Could you check a few things on this model? Use its own coordinates, in mm. A direction names the side the tool comes from. Give positions to 0.01 mm unless a question says otherwise; leave off trailing zeros. Loops run counter-clockwise (first coordinate to the right, second up) from the corner with the lowest first, then second, coordinate; pieces in that order, holes last. Notation, with made-up numbers: M 58,81.5 L 77,81.5 A33 ccw 77,113.5 Z; hole C 18,38 d1. An arc over 180 degrees is marked long. Return JSON: item names as keys, results as strings. Group by question number.
1. If we section it at A-A (z = 33): Write out the boundary of the cut face in (x, y), plus the area to 3 significant figures.
2. Please list where these lines run through material, in increasing order: line 1 (X direction, y = -131.5, z = 76); line 2 (Y direction, x = -170.5, z = 73); line 3 (Y direction, x = -2.5, z = 38.5).
3. For faces 1 (the flat face through (47.709, -113, 50)), 2 (the flat face through (-113, 50.8, 50)), which set-ups out of +Z, -Z, +X, -X, +Y, -Y let a thin tool reach every point of the face, with its end or its side?
4. For pin 1 (5 mm diameter, centred on y = -47, z = 81.5, fed in from -X); pin 2 (8 mm diameter, centred on x = -108, z = 40.5, fed in from -Y); pin 3 (8 mm diameter, centred on y = 23, z = 20.5, fed in from +X), each with a flat end and sliding along its axis, tell me the tip position at first contact or that it passes through.
5. If we section it at C-C (x = -16): Write out the boundary of the cut face in (y, z).
6. If we section it at B-B (y = -64.5): Write out the boundary of the cut face in (x, z).
```python
from build123d import *

# Parameters (mm, degrees)
F1_DEPTH = 101.6
F2_DEPTH = 152.4
F3_DEPTH = 152.4


with BuildPart() as f1:
    # F0 (on Top) → F1 (new body)
    with BuildSketch(Plane.XY):
        with BuildLine():
            Line((50.8, -73.0918422341), (50.8, 0))
            ThreePointArc((50.8, 0), (35.9210244843, 35.9210244843), (0, 50.8))
            Line((0, 50.8), (-76.0997384787, 50.8))
            Line((-76.0997384787, 50.8), (-76.0997384787, 47.9443576366))
            Line((-76.0997384787, 47.9443576366), (-5.2502147954, 47.9443576366))
            ThreePointArc((-5.2502147954, 47.9443576366), (32.074779717, 33.8507856659), (47.7087852046, -2.8556423634))
            Line((47.7087852046, -2.8556423634), (47.7087852046, -73.0918422341))
            Line((47.7087852046, -73.0918422341), (50.8, -73.0918422341))
        make_face()
    extrude(amount=F1_DEPTH)

    # F2 (add): a face of the model
    f2_faces = [f1.faces().sort_by_distance(p)[0] for p in [
        (49.2543926023, -73.0918422341, 50.8),
    ]]
    extrude(f2_faces, amount=F2_DEPTH)

    # F3 (add): a face of the model
    f3_faces = [f1.faces().sort_by_distance(p)[0] for p in [
        (-76.0997384787, 49.3721788183, 50.8),
    ]]
    extrude(f3_faces, amount=F3_DEPTH)


solid = f1.part
```
Answer:
{
 "1": {"outline": "M -228.5,47.94 L -5.25,47.94 A50.8 cw 47.71,-2.86 L 47.71,-225.49 L 50.8,-225.49 L 50.8,0 A50.8 ccw 0,50.8 L -228.5,50.8 Z", "area": "1,640 mm²"},
 "2": {"line 1": "x = 47.71 to 50.8", "line 2": "y = 47.94 to 50.8", "line 3": "y = 47.99 to 50.8"},
 "3": {"face 1": "+Z, -Z, -X, -Y", "face 2": "+Z, -Z, +X, -X, +Y"},
 "4": {"pin 1": "stops at x = 47.71", "pin 2": "stops at y = 47.94", "pin 3": "stops at x = 47.11"},
 "5": {"outline": "M 47.94,0 L 50.8,0 L 50.8,101.6 L 47.94,101.6 Z"},
 "6": {"outline": "M 47.71,0 L 50.8,0 L 50.8,101.6 L 47.71,101.6 Z"}
}
